The listing builds one solid part. Answer for the finished solid, in the listing's coordinates (mm). A direction names the side the tool comes from. Round coordinates to 2 decimals unless told otherwise and drop trailing zeros. Loops run counter-clockwise (first coordinate to the right, second up) from the corner with the lowest first, then second, coordinate; pieces in that order, holes last. Notation, with made-up numbers: (62.25, 24) - (108.25, 24) arc R20 cw to (108.25, 62) - close; hole circle Ø5 at (-23, -11.75). An arc over 180 degrees is marked (long way). Write item = value, one per line. Start each with the question number.
1) Section D-D, the plane x = 9 is taken. Determine the outline of the cut face in (y, z), and give its area (3 significant figures).
2) Straight lines are drawn through the part: line 1 along Y through (x, z) = (0, 7.5); line 2 along Z through (x, y) = (0, 7); line 3 along Y through (x, z) = (-14, 9.75). For each, find the intervals that lie inside material, in ascending order.
3) A tool of negligible diameter and unlimited length cuts with its end or side. For faces 1 (the flat face through (0, 2.825, 11)), 2 (the flat face through (-14.947, 2.472, 4.93)), 3 (the flat face through (-2.472, -14.947, 4.93)), from which of +Z, -Z, +X, -X, +Y, -Y can it reach the whole face along a straight path? Write none if from no direction.
4) Given pin 1 Ø1.5 at (x, z) = (0.5, 12) entering from +Y; pin 2 Ø10 at (x, y) = (6, 11.5) entering from +Z; pin 3 Ø2 at (x, z) = (2.5, 3) entering from -Y, each flat-ended and moving along its own axis, determine where each tip first touches the part or whether it passes through.
5) Section A-A, the plane z = 12 is taken. Determine the outline of the cut face in (x, y) (3 decimals), and give its area (3 significant figures).
6) Section C-C, the plane z = 4.75 is taken. Determine the outline of the cut face in (x, y).
7) For a pull along Y with two mould halves and no side action, classify faces 4 (the cylindrical face through (-16.392, 6.803, 4.93)), 5 (the flat face through (2.2, -2.2, 13)), 6 (the cylindrical face through (-6.78, 16.4, 4.93)) as released by +Y, released by -Y, zero draft, split by the parting line, or undercut.
8) Section B-B, the plane y = -4 is taken. Determine the outline of the cut face in (x, z), and give its area (3 significant figures).
from build123d import *

# Parameters (mm, degrees)
F1_DEPTH = 10
F2_R     = 5
F3_DEPTH = 3
F4_R     = 1.75
F5_DEPTH = 10.001


with BuildPart() as f1:
    # F0 (on Top) → F1 (new body)
    with BuildSketch(Plane.XY):
        with BuildLine():
            Line((-7.971794, 15.117246), (-9.695514, 9.43691))
            Line((-9.695514, 9.43691), (-15.102408, 7.920959))
            ThreePointArc((-15.102408, 7.920959), (-16.401997, 6.78019), (-16.326416, 5.052598))
            Line((-16.326416, 5.052598), (-13.528667, -0.182861))
            Line((-13.528667, -0.182861), (-16.279979, -5.078052))
            ThreePointArc((-16.279979, -5.078052), (-16.392282, -6.803645), (-15.117246, -7.971794))
            Line((-15.117246, -7.971794), (-9.43691, -9.695514))
            Line((-9.43691, -9.695514), (-7.920959, -15.102408))
            ThreePointArc((-7.920959, -15.102408), (-6.78019, -16.401997), (-5.052598, -16.326416))
            Line((-5.052598, -16.326416), (0.182861, -13.528667))
            Line((0.182861, -13.528667), (5.078052, -16.279979))
            ThreePointArc((5.078052, -16.279979), (6.803645, -16.392282), (7.971794, -15.117246))
            Line((7.971794, -15.117246), (9.695514, -9.43691))
            Line((9.695514, -9.43691), (15.102408, -7.920959))
            ThreePointArc((15.102408, -7.920959), (16.401997, -6.78019), (16.326416, -5.052598))
            Line((16.326416, -5.052598), (13.528667, 0.182861))
            Line((13.528667, 0.182861), (16.279979, 5.078052))
            ThreePointArc((16.279979, 5.078052), (16.392282, 6.803645), (15.117246, 7.971794))
            Line((15.117246, 7.971794), (9.43691, 9.695514))
            Line((9.43691, 9.695514), (7.920959, 15.102408))
            ThreePointArc((7.920959, 15.102408), (6.78019, 16.401997), (5.052598, 16.326416))
            Line((5.052598, 16.326416), (-0.182861, 13.528667))
            Line((-0.182861, 13.528667), (-5.078052, 16.279979))
            ThreePointArc((-5.078052, 16.279979), (-6.803645, 16.392282), (-7.971794, 15.117246))
        make_face()
    extrude(amount=F1_DEPTH)

    # F2 (on face) → F3 (join)
    with BuildSketch(Plane.XY.offset(10)):
        Circle(F2_R)
        Polygon((-3.262029, 0), (-1.631015, 2.825), (1.631015, 2.825), (3.262029, 0), (1.631015, -2.825), (-1.631015, -2.825), align=None, mode=Mode.SUBTRACT)
    extrude(amount=F3_DEPTH)

    # F4 (on face) → F5 (cut, through all)
    with BuildSketch(Plane.XY.offset(10)):
        Circle(F4_R)
    extrude(amount=-F5_DEPTH, mode=Mode.SUBTRACT)


solid = f1.part
Geometry check:
q1.outline = (-11.73, 0) - (11.25, 0) - (11.25, 10) - (-11.73, 10) - close
q1.area = 230 mm2
q2.line_1 = -13.63 to -1.75, 1.75 to 13.63
q2.line_2 = 0 to 10
q2.line_3 = -8.31 to -1.02, 0.7 to 8.23
q3.face_1 = +Z
q3.face_2 = +Z, -Z, -X
q3.face_3 = +Z, -Z, -Y
q4.pin_1 = 5
q4.pin_2 = 10
q4.pin_3 = -15.39
q5.outline = circle Ø10 at (0, 0); hole (-3.262, 0) - (-1.631, -2.825) - (1.631, -2.825) - (3.262, 0) - (1.631, 2.825) - (-1.631, 2.825) - close
q5.area = 50.9 mm2
q6.outline = (-16.33, 5.05) - (-13.53, -0.18) - (-16.28, -5.08) arc R2 ccw to (-15.12, -7.97) - (-9.44, -9.7) - (-7.92, -15.1) arc R2 ccw to (-5.05, -16.33) - (0.18, -13.53) - (5.08, -16.28) arc R2 ccw to (7.97, -15.12) - (9.7, -9.44) - (15.1, -7.92) arc R2 ccw to (16.33, -5.05) - (13.53, 0.18) - (16.28, 5.08) arc R2 ccw to (15.12, 7.97) - (9.44, 9.7) - (7.92, 15.1) arc R2 ccw to (5.05, 16.33) - (-0.18, 13.53) - (-5.08, 16.28) arc R2 ccw to (-7.97, 15.12) - (-9.7, 9.44) - (-15.1, 7.92) arc R2 ccw to start; hole circle Ø3.5 at (0, 0)
q7.face_4 = undercut
q7.face_5 = zero draft
q7.face_6 = released by +Y
q8.outline = (-15.67, 0) - (15.76, 0) - (15.76, 10) - (3, 10) - (3, 13) - (-3, 13) - (-3, 10) - (-15.67, 10) - close
q8.area = 332 mm2
